Part model, mm, in its own coordinate system. A direction names the side the tool comes from. Coordinates: 2 decimals unless noted, no trailing zeros. Order: outer loops, then holes, each group sorted by start corner. A loop starts at its lowest first (then second) coordinate and runs counter-clockwise, first axis right, second up.
1) Cut at B-B (x = 40). List the corners of the cut face in (y, z), and give its area (3 significant figures).
2) Mould opens along Z. For faces 1 (the flat face through (90, 3, -55)), 2 (the flat face through (12.93, 3.296, -355.355)), 3 (the flat face through (52, 0, -241)) say: +Z half, -Z half, draft (parallel to the pull), parting line (faces both ways), or undercut.
3) Tool access for faces 4 (the flat face through (111.7, 3.2, -368.2)), 5 (the flat face through (13.05, 3.3, -340.35)), 6 (the flat face through (52, 6.5, -241)): list every direction of +Z, -Z, +X, -X, +Y, -Y with a clear straight run to the whole face (end or side of a thin tool).
4) Pin check, flat tips, straight feed: pin 1 Ø1 at (x, z) = (97.5, -411) entering from -Y; pin 2 Ø2 at (x, y) = (14, 2.5) entering from -Z; pin 3 Ø3 at (x, y) = (64.5, 3.5) entering from -Z; pin 4 Ø1.6 at (y, z) = (5, -239.5) entering from -X. Stop position of each tip, or through.
5) Wall check: L1, parallel to X at y = 3, z = -240; L2, parallel to Z at x = 9.5, y = 3; L3, parallel to X at y = 4.5, z = -303. Give the ranges that are in metal, low to high.
6) Cut at C-C (z = -316). List the corners of the cut face in (x, y).
7) Cut at A-A (z = -461). List the corners of the cut face in (x, y).
Autodesk Inventor part; units mm, degrees
ref_plane "YZ Plane" through (0, 0, 0) normal (1, 0, 0) x (0, 1, 0)
ref_plane "XZ Plane" through (0, 0, 0) normal (0, 1, 0) x (-1, 0, 0)
ref_plane "XY Plane" through (0, 0, 0) normal (0, 0, 1) x (1, 0, 0)
sketch "Sketch1" plane through (0, 0, 0) normal (0, 1, 0) x (-1, 0, 0)
  line L0 (0, 0) -> (0, -489)
  line L1 (0, -489) -> (-30.25, -489)
  line L2 (-30.25, -489) -> (-30.25, -439)
  line L3 (-30.25, -439) -> (-112.25, -439)
  line L4 (-112.25, -439) -> (-112.25, -489)
  line L5 (-112.25, -489) -> (-142.5, -489)
  line L6 (-142.5, -489) -> (-142.5, -399)
  line L7 (-142.5, -399) -> (-80, -336.5)
  line L8 (-80, -336.5) -> (-80, -65)
  line L9 (-80, -65) -> (-100, -45)
  line L10 (-100, -45) -> (-100, 0)
  line L11 (-100, 0) -> (0, 0)
  dimension "d0" = 135
  dimension "d1" = 100
  dimension "d2" = 489
  dimension "d3" = 45
  dimension "d4" = 20
  dimension "d5" = 30.25
  dimension "d6" = 50
  dimension "d7" = 82
  dimension "d8" = 40
extrude "Extrusion1" add sketch "Sketch1" along normal blind 6.5
sketch "Sketch2" plane through (0, 6.5, 0) normal (0, 1, 0) x (1, 0, 0)
  line L0 (0, 0) -> (100, 0)
  line L1 (30.25, 489) -> (0, 489)
  line L2 (0, 489) -> (0, 0)
  line L3 (16.3, 425.75) -> (16.3, 421.25)
  line L4 (0, 421.25) -> (0, 425.75)
  line L5 (5, 428.25) -> (12.3, 428.25)
  line L6 (12.3, 418.75) -> (5, 418.75)
  line L7 (0, 425.75) -> (5, 425.75)
  line L8 (12.3, 425.75) -> (16.3, 425.75)
  line L9 (16.3, 421.25) -> (12.3, 421.25)
  line L10 (5, 421.25) -> (0, 421.25)
  line L11 (5, 418.75) -> (5, 421.25)
  line L12 (5, 425.75) -> (5, 428.25)
  line L13 (12.3, 428.25) -> (12.3, 425.75)
  line L14 (12.3, 421.25) -> (12.3, 418.75)
  line L15 (16.3, 246.75) -> (16.3, 242.25)
  line L16 (0, 242.25) -> (0, 246.75)
  line L17 (5, 249.25) -> (12.3, 249.25)
  line L18 (12.3, 239.75) -> (5, 239.75)
  line L19 (0, 246.75) -> (5, 246.75)
  line L20 (12.3, 246.75) -> (16.3, 246.75)
  line L21 (16.3, 242.25) -> (12.3, 242.25)
  line L22 (5, 242.25) -> (0, 242.25)
  line L23 (5, 239.75) -> (5, 242.25)
  line L24 (5, 246.75) -> (5, 249.25)
  line L25 (12.3, 249.25) -> (12.3, 246.75)
  line L26 (12.3, 242.25) -> (12.3, 239.75)
  line L27 (16.3, 67.75) -> (16.3, 63.25)
  line L28 (0, 63.25) -> (0, 67.75)
  line L29 (5, 70.25) -> (12.3, 70.25)
  line L30 (12.3, 60.75) -> (5, 60.75)
  line L31 (0, 67.75) -> (5, 67.75)
  line L32 (12.3, 67.75) -> (16.3, 67.75)
  line L33 (16.3, 63.25) -> (12.3, 63.25)
  line L34 (5, 63.25) -> (0, 63.25)
  line L35 (5, 60.75) -> (5, 63.25)
  line L36 (5, 67.75) -> (5, 70.25)
  line L37 (12.3, 70.25) -> (12.3, 67.75)
  line L38 (12.3, 63.25) -> (12.3, 60.75)
  line L39 (8.65, 418.75) -> (8.65, 249.25) construction
  line L40 (8.65, 239.75) -> (8.65, 70.25) construction
  point P0 (16.3, 423.5)
  point P1 (16.3, 244.5)
  point P2 (16.3, 65.5)
  dimension "d11" = 4.5
  dimension "d12" = 5
  dimension "d13" = 4
  dimension "d14" = 7.3
  dimension "d15" = 2.5
  dimension "d16" = 4.5
  dimension "d17" = 5
  dimension "d18" = 4
  dimension "d19" = 7.3
  dimension "d20" = 2.5
  dimension "d21" = 4.5
  dimension "d22" = 5
  dimension "d23" = 4
  dimension "d24" = 7.3
  dimension "d25" = 2.5
  dimension "d26" = 65.5
  dimension "d27" = 65.5
extrude "Extrusion2" cut sketch "Sketch2" against normal through all
sketch "Sketch3" plane through (0, 6.5, 0) normal (0, 1, 0) x (1, 0, 0)
  line L0 (0, 242.25) -> (0, 67.75)
  line L1 (16.3, 67.75) -> (16.3, 63.25)
  line L2 (0, 63.25) -> (0, 0)
  line L3 (0, 489) -> (0, 425.75)
  line L4 (16.3, 425.75) -> (16.3, 421.25)
  line L5 (0, 421.25) -> (0, 246.75)
  line L6 (16.3, 246.75) -> (16.3, 242.25)
  line L7 (0, 439) -> (-4.5, 439)
  line L8 (-6.5, 437) -> (-6.5, 433)
  line L9 (-4.5, 431) -> (0, 431)
  line L10 (0, 431) -> (0, 439)
  line L11 (0, 416) -> (-4.5, 416)
  line L12 (-6.5, 414) -> (-6.5, 410)
  line L13 (-4.5, 408) -> (0, 408)
  line L14 (0, 408) -> (0, 416)
  line L15 (0, 260) -> (-4.5, 260)
  line L16 (-6.5, 258) -> (-6.5, 254)
  line L17 (-4.5, 252) -> (0, 252)
  line L18 (0, 252) -> (0, 260)
  line L19 (0, 237) -> (-4.5, 237)
  line L20 (-6.5, 235) -> (-6.5, 231)
  line L21 (-4.5, 229) -> (0, 229)
  line L22 (0, 229) -> (0, 237)
  line L23 (0, 81) -> (-4.5, 81)
  line L24 (-6.5, 79) -> (-6.5, 75)
  line L25 (-4.5, 73) -> (0, 73)
  line L26 (0, 73) -> (0, 81)
  line L27 (0, 58) -> (-4.5, 58)
  line L28 (-6.5, 56) -> (-6.5, 52)
  line L29 (-4.5, 50) -> (0, 50)
  line L30 (0, 50) -> (0, 58)
  arc A0 (-4.5, 439) -> (-6.5, 437) centre (-4.5, 437) ccw
  arc A1 (-6.5, 433) -> (-4.5, 431) centre (-4.5, 433) ccw
  arc A2 (-4.5, 416) -> (-6.5, 414) centre (-4.5, 414) ccw
  arc A3 (-6.5, 410) -> (-4.5, 408) centre (-4.5, 410) ccw
  arc A4 (-4.5, 260) -> (-6.5, 258) centre (-4.5, 258) ccw
  arc A5 (-6.5, 254) -> (-4.5, 252) centre (-4.5, 254) ccw
  arc A6 (-4.5, 237) -> (-6.5, 235) centre (-4.5, 235) ccw
  arc A7 (-6.5, 231) -> (-4.5, 229) centre (-4.5, 231) ccw
  arc A8 (-4.5, 81) -> (-6.5, 79) centre (-4.5, 79) ccw
  arc A9 (-6.5, 75) -> (-4.5, 73) centre (-4.5, 75) ccw
  arc A10 (-4.5, 58) -> (-6.5, 56) centre (-4.5, 56) ccw
  arc A11 (-6.5, 52) -> (-4.5, 50) centre (-4.5, 52) ccw
  point P0 (16.3, 423.5)
  point P1 (16.3, 244.5)
  point P2 (16.3, 65.5)
  dimension "d30" = 2
  dimension "d31" = 8
  dimension "d32" = 8
  dimension "d33" = 15
  dimension "d34" = 8
  dimension "d35" = 8
  dimension "d36" = 15
  dimension "d37" = 8
  dimension "d38" = 8
  dimension "d39" = 15
  dimension "d40" = 7.5
  dimension "d41" = 7.5
  dimension "d42" = 7.5
  dimension "d43" = 6.5
extrude "Extrusion3" add sketch "Sketch3" against normal blind 6.5
sketch "Sketch4" plane through (0, 6.5, 0) normal (0, 1, 0) x (1, 0, 0)
  line L0 (0, 0) -> (100, 0)
  line L1 (100, 0) -> (100, 45)
  line L2 (142.5, 399) -> (142.5, 489)
  line L3 (142.5, 489) -> (112.25, 489)
  line L4 (77, 0) -> (85, 0)
  line L5 (85, 0) -> (85, -4.5)
  line L6 (83, -6.5) -> (79, -6.5)
  line L7 (77, -4.5) -> (77, 0)
  line L8 (124.5, 489) -> (132.5, 489)
  line L9 (132.5, 489) -> (132.5, 493.5)
  line L10 (130.5, 495.5) -> (126.5, 495.5)
  line L11 (124.5, 493.5) -> (124.5, 489)
  arc A0 (126.5, 495.5) -> (124.5, 493.5) centre (126.5, 493.5) ccw
  arc A1 (132.5, 493.5) -> (130.5, 495.5) centre (130.5, 493.5) ccw
  arc A2 (83, -6.5) -> (85, -4.5) centre (83, -4.5) ccw
  arc A3 (77, -4.5) -> (79, -6.5) centre (79, -4.5) ccw
  dimension "d46" = 2
  dimension "d47" = 8
  dimension "d48" = 6.5
  dimension "d49" = 15
  dimension "d50" = 8
  dimension "d51" = 6.5
  dimension "d52" = 10
extrude "Extrusion4" add sketch "Sketch4" against normal blind 6.5
sketch "Sketch5" plane through (0, 6.5, 0) normal (0, 1, 0) x (1, 0, 0)
  line L0 (30.25, 489) -> (0, 489)
  line L1 (0, 408) -> (0, 260)
  line L2 (8.6603, 332.75) -> (0, 332.75)
  line L3 (0, 362.75) -> (8.6603, 362.75)
  line L4 (8.6603, 362.75) -> (17.3205, 347.75)
  line L5 (17.3205, 347.75) -> (8.6603, 332.75)
  line L6 (0, 362.75) -> (0, 332.75)
  point P0 (0, 347.75)
  dimension "d55" = 30
  dimension "d56" = 156.25
extrude "Extrusion5" cut sketch "Sketch5" against normal through all
chamfer "Chamfer1" distance 4 angle 45 1 edges at (0, 3.25, 0)
equation "\"d32\" = d31"
equation "\"d34\" = d32"
equation "\"d35\" = d34"
equation "\"d36\" = d33"
equation "\"d37\" = d35"
equation "\"d38\" = d37"
equation "\"d39\" = d36"
equation "\"d50\" = d47"
equation "\"d51\" = d48"
properties part number "inner_brace_left" material "Plywood, Finish"
Geometry check:
1. outline: (0, -439) - (6.5, -439) - (6.5, 0) - (0, 0) - close
1. area: 2,850 mm2
2. face 1: undercut
2. face 2: undercut
2. face 3: draft
3. face 4: +X, +Y, -Y
3. face 5: -X, +Y, -Y
3. face 6: +Z, -Z, +X, -X, +Y
4. pin 1: stops at y = 0
4. pin 2: stops at z = -489
4. pin 3: stops at z = -439
4. pin 4: stops at x = 0
5. L1: x = 0 to 5, 12.3 to 80
5. L2: z = -489 to -428.25, -418.75 to -361.3, -334.2 to -249.25, -239.75 to -70.25, -60.75 to 0
5. L3: x = 0 to 80
6. outline: (0, 0) - (80, 0) - (80, 6.5) - (0, 6.5) - close
7. outline: (0, 0) - (30.25, 0) - (30.25, 6.5) - (0, 6.5) - close; (112.25, 0) - (142.5, 0) - (142.5, 6.5) - (112.25, 6.5) - close
